Here's how the part is built. I have some questions about the finished solid (model axes, mm). A direction names the side the tool comes from. Coordinates: 2 decimals unless noted, no trailing zeros. Write each loop counter-clockwise with the first axis right and the second up, starting at its lowest first coordinate (ties: lowest second). Pieces come first, ordered by that corner, then holes.
(1) For pin 1 Ø16 at (y, z) = (-173.5, 216.5) entering from +X; pin 2 Ø8 at (x, z) = (-23.5, 258) entering from -Y, each with a flat end and sliding along its axis, tell me the tip position at first contact or that it passes through.
(2) Which directions (+Z, -Z, +X, -X, +Y, -Y) give clear straight access to the entire face, cutting with the end or side of a thin tool? Please do faces 5 (the flat face through (-30, -89, 150)), 6 (the flat face through (-30, -170, 224)), 7 (the flat face through (-30, -10, 195)).
(3) Please list where these lines run through material, in increasing order: probe 1 along Z at (x, y) = (-22.5, -10); probe 2 along Y at (x, z) = (-26, 225); probe 3 along X at (y, z) = (-166, 263.5).
(4) Imagine slicing it at A-A, the plane z = 255. List the corners of the cut face in (x, y) for me, plus the area to 3 significant figures.
(5) Thinking about a two-plate mould opening in Y: for faces 1 (the flat face through (-30, 0, 226)), 2 (the cylindrical face through (-24.9, -7.2, 197.1)), 3 (the flat face through (-30, -10, 225)), 4 (the flat face through (-20, -79, 224)), which applies, released by +Y, released by -Y, zero draft, split by the parting line, or undercut?
(6) Imagine slicing it at B-B, the plane z = 180.5. List the corners of the cut face in (x, y) for me, plus the area to 3 significant figures.
```python
from build123d import *

# Parameters (mm, degrees)
F0_W     = 180
F0_H     = 150
F1_DEPTH = 20
F2_R     = 3.5
F3_DEPTH = 10
F4_W     = 20
F4_H     = 150
F5_DEPTH = 10
F6_ANGLE = 180
F7_ANGLE = -90
F8_ANGLE = 180


with BuildPart() as f1:
    # F0 (on Front) → F1 (new body)
    with BuildSketch(Plane.XZ):
        with Locations((90, 75)):
            Rectangle(F0_W, F0_H)
    extrude(amount=F1_DEPTH)

    # F2 (on face) → F3 (cut)
    with BuildSketch(Plane.XZ.offset(20)):
        with Locations((10, 75)):
            Circle(F2_R)
        with Locations((10, 105)):
            Circle(F2_R)
        with Locations((10, 45)):
            Circle(F2_R)
    extrude(amount=-F3_DEPTH, mode=Mode.SUBTRACT)

    # F4 (on face) → F5 (cut)
    with BuildSketch(Plane.XZ.offset(20)):
        with Locations((170, 75)):
            Rectangle(F4_W, F4_H)
    extrude(amount=-F5_DEPTH, mode=Mode.SUBTRACT)


with BuildPart() as f1_1:
    # F6: moved
    add(f1.part.rotate(Axis((90, 0, 150), (1, 0, 0)), F6_ANGLE))


with BuildPart() as f1_2:
    # F7: moved
    add(f1_1.part.rotate(Axis((0, 0, 225), (0, 0, -1)), F7_ANGLE))


with BuildPart() as f1_3:
    # F8: moved
    add(f1_2.part.rotate(Axis((-20, 0, 225), (0, 0, -1)), F8_ANGLE))


solid = f1_3.part
```
Recorded:
1. pin 1: stops at x = -30
1. pin 2: stops at y = -160
2. face 5: -Z, +X, -X, +Y, -Y
2. face 6: +Z, -Z, +X, -Y
2. face 7: +X
3. probe 1: z = 150 to 191.5, 198.5 to 221.5, 228.5 to 251.5, 258.5 to 300
3. probe 2: y = -160 to -13.5, -6.5 to 0
3. probe 3: x = -40 to -30
4. outline: (-40, -180) - (-30, -180) - (-30, -160) - (-20, -160) - (-20, -13.5) - (-30, -13.5) - (-30, -6.5) - (-20, -6.5) - (-20, 0) - (-40, 0) - close
4. area: 3,330 mm2
5. face 1: released by +Y
5. face 2: undercut
5. face 3: undercut
5. face 4: zero draft
6. outline: (-40, -180) - (-30, -180) - (-30, -160) - (-20, -160) - (-20, 0) - (-40, 0) - close
6. area: 3,400 mm2
